Autodesk Inventor part; units mm, degrees
ref_plane "YZ Plane" through (0, 0, 0) normal (1, 0, 0) x (0, 1, 0)
ref_plane "XZ Plane" through (0, 0, 0) normal (0, 1, 0) x (-1, 0, 0)
ref_plane "XY Plane" through (0, 0, 0) normal (0, 0, 1) x (1, 0, 0)
sketch "Sketch1" plane through (0, 0, 0) normal (0, 0, 1) x (1, 0, 0)
  line L0 (0, 0) -> (0, 3.175)
  line L1 (0, 0) -> (25.4, 0)
  line L2 (25.4, 0) -> (25.4, 3.175)
  line L3 (25.4, 3.175) -> (13.0737, 49.1772)
  line L4 (13.0737, 49.1772) -> (10.0069, 48.3555)
  line L5 (10.0069, 48.3555) -> (22.113, 3.175)
  line L6 (0, 3.175) -> (22.113, 3.175)
  dimension "d0" = 3.175
  dimension "d1" = 25.4
  dimension "d3" = 3.175
  dimension "d4" = 75
  dimension "d5" = 47.625
extrude "Extrusion1" add sketch "Sketch1" along normal blind 28.575
sketch "Sketch2" plane through (10.0069, 48.3555, 0) normal (-0.9659, -0.2588, 0) x (0, 0, 1)
  line L0 (28.575, -46.7743) -> (28.575, 0)
  line L1 (0, 0) -> (28.575, 0)
  circle A0 centre (14.2875, -14.2875) radius 9.525
  point P0 (0, -44.1178)
  dimension "d8" = 19.05
  dimension "d9" = 14.2875
  dimension "d10" = 14.2875
extrude "Extrusion2" cut sketch "Sketch2" against normal blind 28.575
fillet "Fillet1" radius 3.175 1 edges at (25.4, 3.175, 14.2875)
equation "\"d3\" = d0"
equation "\"d10\" = d9"
properties part number "bunny throw piston bracket"
Can you work these out from the model? Positions are in its coordinate system, mm. A direction names the side the tool comes from. Coordinates: 2 decimals unless noted, no trailing zeros. Write each loop counter-clockwise with the first axis right and the second up, starting at its lowest first coordinate (ties: lowest second). Pieces come first, ordered by that corner, then holes.
Q1. Which directions (+Z, -Z, +X, -X, +Y, -Y) give clear straight access to the entire face, cutting with the end or side of a thin tool? Please do faces 4 (the face through (11, 3.175, 14)), 5 (the face through (19, 19, 0)).
Results found:
face 4: +Z, -Z, -X
face 5: -Z, +X, -X, +Y, -Y
Q2. For P1, Ø5, axis at y = 20, z = 13.5, coming from the +X side; P2, Ø2, axis at y = 32.5, z = 25, coming from the -X side; P3, Ø6, axis at x = 6, z = 21.5, coming from the +Y side (3 decimals), each with a flat end and sliding along its axis, tell me the tip position at first contact or that it passes through.
Results found:
P1: stops at x = 21.56
P2: stops at x = 13.99
P3: stops at y = 3.175
Q3. If we mould it in two halves opening along Z, with no side actions, what happens to faces 1 (the face through (17.32, 21.06, 14.09)), 2 (the face through (14.476, 37.724, 23.373)), 3 (the face through (19, 19, 28.575))? For each: +Z half, -Z half, draft (parallel to the pull), parting line (faces both ways), or undercut.
Results found:
face 1: draft
face 2: undercut
face 3: +Z half
Q4. Imagine slicing it at C-C, the plane x = 4. List the corners of the cut face in (y, z) for me (3 decimals).
Results found:
outline: (0, 0) - (3.175, 0) - (3.175, 28.575) - (0, 28.575) - close
Q5. Please list where these lines run through material, in increasing order: L1, parallel to Y at x = 8.25, z = 22.25 (3 decimals); L2, parallel to Y at x = 12.25, z = 7.25 (1 decimal); L3, parallel to X at y = 10.5, z = 7.75.
Results found:
L1: y = 0 to 3.175
L2: y = 0 to 3.2, 40.8 to 49
L3: x = 20.15 to 23.44
